Could you check a few things on this drawing? It's one solid part, dimensions in mm from its lowest x, y, z. A direction names the side the tool comes from. Coordinates: 2 decimals unless noted, no trailing zeros. Order: outer loops, then holes, each group sorted by start corner. A loop starts at its lowest first (then second) coordinate and runs counter-clockwise, first axis right, second up. Notation, with made-up numbers: (-1, 61.25) -> (14, 61.25) arc R7 cw to (14, 67.25) -> close; hole circle Ø1 at (-13.5, -13.75). An arc over 180 degrees is marked (long way). Use a Markdown table: item, result. Add a question column.
1. Suppose I cut it at C-C, the plane x = 13.97. List the corners of the cut face in (y, z) for me (3 decimals).
2. We'd pull the mould along Y, two halves only. Please class the marked faces 4, 5 and 6: pulls with the +Y half, pulls with the -Y half, needs draft (parallel to the pull), parting line crosses it, or undercut.
3. If I drill on line 1 along Y through (x, z) = (13.97, 1.5) (3 decimals); line 2 along Y through (x, z) = (10, 24); line 3 along Z through (x, y) = (11.5, 53.5), over which ranges is the centre line in solid material (lowest first)? Write a range as from..to.
4. For the marked faces 1, 2 and 3, which set-ups out of +Z, -Z, +X, -X, +Y, -Y let a thin tool reach every point of the face, with its end or its side?
5. Suppose I cut it at B-B, the plane x = 4.5. List the corners of the cut face in (y, z) for me.
6. Suppose I cut it at D-D, the plane x = 17.25. List the corners of the cut face in (y, z) for me, then the cut area to 3 significant figures.
7. For pin 1 Ø6.5 at (x, z) = (13.5, 20) entering from +Y; pin 2 Ø12 at (x, y) = (23.5, 30.5) entering from -Z; pin 3 Ø8 at (y, z) = (65.5, 10.5) entering from -X; pin 4 Ø4 at (x, y) = (13.97, 76.835) entering from -Z, each with a flat end and sliding along its axis, tell me the tip position at first contact or that it passes through.
8. Suppose I cut it at A-A, the plane z = 12.5. List the corners of the cut face in (x, y) for me.
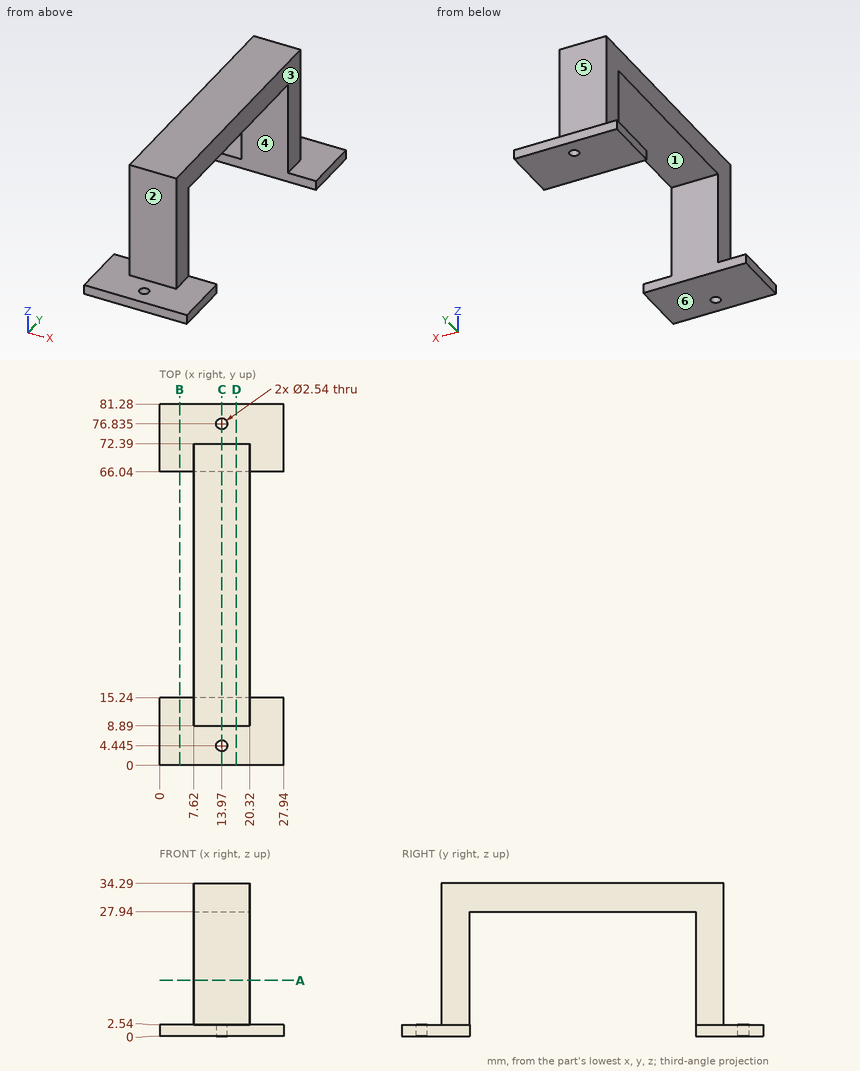
Worked out:
| question | item | result |
|---|---|---|
| 1 | outline | (0, 0) -> (3.175, 0) -> (3.175, 2.54) -> (0, 2.54) -> close; (5.715, 0) -> (15.24, 0) -> (15.24, 27.94) -> (66.04, 27.94) -> (66.04, 0) -> (75.565, 0) -> (75.565, 2.54) -> (72.39, 2.54) -> (72.39, 34.29) -> (8.89, 34.29) -> (8.89, 2.54) -> (5.715, 2.54) -> close; (78.105, 0) -> (81.28, 0) -> (81.28, 2.54) -> (78.105, 2.54) -> close |
| 2 | face 4 | undercut |
| 2 | face 5 | pulls with the +Y half |
| 2 | face 6 | needs draft |
| 3 | line 1 | y = 0..3.175, 5.715..15.24, 66.04..75.565, 78.105..81.28 |
| 3 | line 2 | y = 8.89..15.24, 66.04..72.39 |
| 3 | line 3 | z = 27.94..34.29 |
| 4 | face 1 | -Z, +X, -X |
| 4 | face 2 | +Z, +X, -X, -Y |
| 4 | face 3 | +Z, +X, +Y, -Y |
| 5 | outline | (0, 0) -> (15.24, 0) -> (15.24, 2.54) -> (0, 2.54) -> close; (66.04, 0) -> (81.28, 0) -> (81.28, 2.54) -> (66.04, 2.54) -> close |
| 6 | outline | (0, 0) -> (15.24, 0) -> (15.24, 27.94) -> (66.04, 27.94) -> (66.04, 0) -> (81.28, 0) -> (81.28, 2.54) -> (72.39, 2.54) -> (72.39, 34.29) -> (8.89, 34.29) -> (8.89, 2.54) -> (0, 2.54) -> close |
| 6 | area | 803 mm² |
| 7 | pin 1 | stops at y = 72.39 |
| 7 | pin 2 | stops at z = 27.94 |
| 7 | pin 3 | stops at x = 7.62 |
| 7 | pin 4 | stops at z = 0 |
| 8 | outline | (7.62, 8.89) -> (20.32, 8.89) -> (20.32, 15.24) -> (7.62, 15.24) -> close; (7.62, 66.04) -> (20.32, 66.04) -> (20.32, 72.39) -> (7.62, 72.39) -> close |
